Here's the drawing with two shaded views (mm, measured from the low corner). I have some questions. Round coordinates to 2 decimals unless told otherwise and drop trailing zeros. Order: outer loops, then holes, each group sorted by start corner. A loop starts at its lowest first (then second) coordinate and runs counter-clockwise, first axis right, second up. Notation, with made-up numbers: (56, -15.75) -> (112, -15.75) arc R26 cw to (112, 17.25) -> close; hole circle Ø10 at (69, 79.5). An arc over 180 degrees is marked (long way). Use a Markdown table: item, result. Add a question column.
Q1. I need wall thicknesses on line 1 along Y through (x, z) = (124.5, 5.25); line 2 along Y through (x, z) = (55, 1). Which ranges of each line are inside material? Lowest first, please. Write a range as [from, to].
Q2. I'm going to push flat-ended pins straight in: pin 1 Ø3 at (x, z) = (125.5, 5) entering from +Y; pin 2 Ø1 at (x, z) = (102.5, 3.5) entering from +Y; pin 3 Ø3 at (x, z) = (54, 5) entering from +Y. Where does each tip first touch, or does it pass through?
Q3. If we section it at B-B on x = 122: List the corners of the cut face in (y, z) for me, plus the area to 3 significant figures.
Q4. If we section it at C-C on x = 84: List the corners of the cut face in (y, z) for me, plus the area to 3 significant figures.
Q5. If we section it at A-A on z = 2.5: List the corners of the cut face in (x, y) for me.
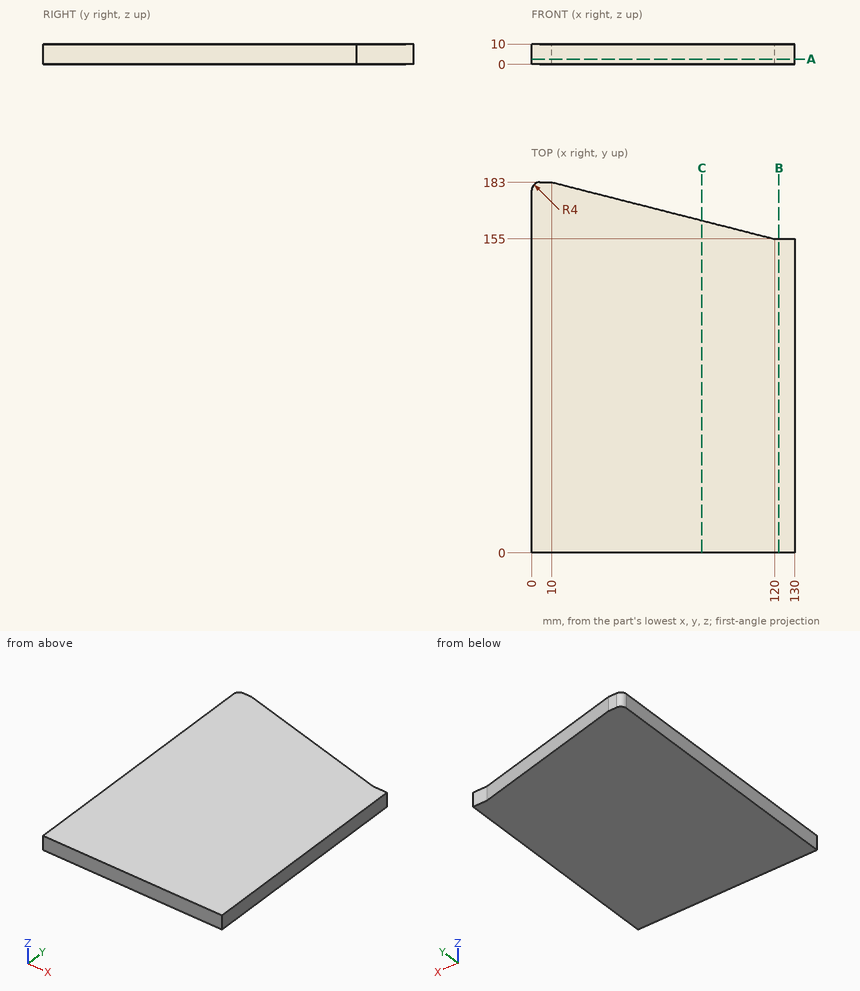
Answer below:
| question | item | result |
|---|---|---|
| 1 | line 1 | [0, 155] |
| 1 | line 2 | [0, 171.55] |
| 2 | pin 1 | y = 155 |
| 2 | pin 2 | y = 159.58 |
| 2 | pin 3 | y = 172.18 |
| 3 | outline | (0, 0) -> (155, 0) -> (155, 10) -> (0, 10) -> close |
| 3 | area | 1,550 mm² |
| 4 | outline | (0, 0) -> (164.16, 0) -> (164.16, 10) -> (0, 10) -> close |
| 4 | area | 1,640 mm² |
| 5 | outline | (0, 0) -> (130, 0) -> (130, 155) -> (120, 155) -> (10, 183) -> (4, 183) arc R4 ccw to (0, 179) -> close |
